```python
from build123d import *

# Parameters (mm, degrees)
BOSS_EXTRUDE1_DEPTH = 5.5118
SKETCH2_R           = 5.08
CUT_EXTRUDE1_DEPTH  = 2.286
BOSS_EXTRUDE2_DEPTH = 4.6228


with BuildPart() as part:
    # Sketch1 → Boss-Extrude1 (new body)
    with BuildSketch(Plane(origin=(0, 0, 0), x_dir=(1, 0, 0), z_dir=(0, 1, 0))):
        with BuildLine():
            ThreePointArc((20.407631134, 9.827266142), (20.718157649, 9.399980692), (20.828, 8.88332391))
            Line((20.828, 8.88332391), (20.828, -4.0386))
            Line((20.828, -4.0386), (24.257, -4.0386))
            Line((24.257, -4.0386), (24.257, -8.9916))
            ThreePointArc((24.257, -8.9916), (23.95942049, -9.71002049), (23.241, -10.0076))
            Line((23.241, -10.0076), (22.352, -10.0076))
            ThreePointArc((22.352, -10.0076), (21.274369265, -10.453969265), (20.828, -11.5316))
            Line((20.828, -11.5316), (20.828, -18.5166))
            Line((20.828, -18.5166), (-20.828, -18.5166))
            Line((-20.828, -18.5166), (-20.828, -11.5316))
            ThreePointArc((-20.828, -11.5316), (-21.274369265, -10.453969265), (-22.352, -10.0076))
            Line((-22.352, -10.0076), (-23.241, -10.0076))
            ThreePointArc((-23.241, -10.0076), (-23.95942049, -9.71002049), (-24.257, -8.9916))
            Line((-24.257, -8.9916), (-24.257, -4.0386))
            Line((-24.257, -4.0386), (-20.828, -4.0386))
            Line((-20.828, -4.0386), (-20.828, 8.88332391))
            ThreePointArc((-20.828, 8.88332391), (-20.718157649, 9.399980692), (-20.407631134, 9.827266142))
            Line((-20.407631134, 9.827266142), (-11.478262268, 17.864484463))
            ThreePointArc((-11.478262268, 17.864484463), (-10.689047654, 18.347973709), (-9.779, 18.5166))
            Line((-9.779, 18.5166), (9.779, 18.5166))
            ThreePointArc((9.779, 18.5166), (10.689047654, 18.347973709), (11.478262268, 17.864484463))
            Line((11.478262268, 17.864484463), (20.407631134, 9.827266142))
        make_face()
    extrude(amount=BOSS_EXTRUDE1_DEPTH)

    # Sketch2 → Cut-Extrude1 (cut)
    with BuildSketch(Plane(origin=(0, 5.5118, 0), x_dir=(1, 0, 0), z_dir=(0, 1, 0))):
        with Locations(Location((-9.9695, 0.7366, 0), (0, 0, 270))):
            Circle(SKETCH2_R)
        with Locations(Location((9.9695, 0.7366, 0), (0, 0, 270))):
            Circle(SKETCH2_R)
    extrude(amount=-CUT_EXTRUDE1_DEPTH, mode=Mode.SUBTRACT)

    # Sketch3 → Boss-Extrude2 (add)
    with BuildSketch(Plane.XZ):
        with BuildLine():
            Line((10.795, -17.2466), (-10.795, -17.2466))
            Line((-10.795, -17.2466), (-20.045633867, -8.920214887))
            Line((-20.045633867, -8.920214887), (-20.045633867, 11.4554))
            ThreePointArc((-20.045633867, 11.4554), (0, 12.967759921), (20.045633867, 11.4554))
            Line((20.045633867, 11.4554), (20.045633867, -8.920214887))
            Line((20.045633867, -8.920214887), (10.795, -17.2466))
        make_face()
    extrude(amount=BOSS_EXTRUDE2_DEPTH)


solid = part.part
```
Build history of the part. All positions in model axes, mm. A direction names the side the tool comes from. Round coordinates to 2 decimals unless told otherwise and drop trailing zeros. Write each loop counter-clockwise with the first axis right and the second up, starting at its lowest first coordinate (ties: lowest second). Pieces come first, ordered by that corner, then holes. Notation, with made-up numbers: (42, -29) -> (100, -29) arc R14 ccw to (100, -13) -> close; hole circle Ø7 at (67, 11.25). An arc over 180 degrees is marked (long way). Put each result on its own line as item: value.
Item 1: Slice it at A-A, the plane y = -3.25. Give the cut face in (x, z) (3 decimals).
Here are the results:
outline: (-20.046, -8.92) -> (-10.795, -17.247) -> (10.795, -17.247) -> (20.046, -8.92) -> (20.046, 11.455) arc R133.604 ccw to (-20.046, 11.455) -> close
Item 2: Slice it at C-C, the plane z = -15.5. Give the cut face in (x, y), plus the area to 3 significant figures.
Here are the results:
outline: (-14.11, 0) -> (-12.74, 0) -> (-12.74, -4.62) -> (12.74, -4.62) -> (12.74, 0) -> (14.11, 0) -> (14.11, 5.51) -> (-14.11, 5.51) -> close
area: 273 mm^2
Item 3: Wall check: probe 1 along X at (y, z) = (4.5, -5); probe 2 along Y at (x, z) = (-20.5, 6); probe 3 along X at (y, z) = (-0.5, 9). Give the ranges that are in metal, low to high. Write a range as from..to.
Here are the results:
probe 1: x = -20.83..-12.73, -7.21..7.21, 12.73..20.83
probe 2: y = 0..5.51
probe 3: x = -20.05..20.05
Item 4: Slice it at D-D, the plane y = 4. Give the cut face in (x, z), plus the area to 3 significant figures.
Here are the results:
outline: (-24.26, 4.04) -> (-20.83, 4.04) -> (-20.83, -8.88) arc R1.27 ccw to (-20.41, -9.83) -> (-11.48, -17.86) arc R2.54 ccw to (-9.78, -18.52) -> (9.78, -18.52) arc R2.54 ccw to (11.48, -17.86) -> (20.41, -9.83) arc R1.27 ccw to (20.83, -8.88) -> (20.83, 4.04) -> (24.26, 4.04) -> (24.26, 8.99) arc R1.02 ccw to (23.24, 10.01) -> (22.35, 10.01) arc R1.52 cw to (20.83, 11.53) -> (20.83, 18.52) -> (-20.83, 18.52) -> (-20.83, 11.53) arc R1.52 cw to (-22.35, 10.01) -> (-23.24, 10.01) arc R1.02 ccw to (-24.26, 8.99) -> close; hole circle Ø10.16 at (-9.97, -0.74); hole circle Ø10.16 at (9.97, -0.74)
area: 1,330 mm^2
Item 5: Slice it at B-B, the plane x = -5.5. Give the cut face in (y, z).
Here are the results:
outline: (-4.62, -17.25) -> (0, -17.25) -> (0, -18.52) -> (5.51, -18.52) -> (5.51, -3.15) -> (3.23, -3.15) -> (3.23, 1.68) -> (5.51, 1.68) -> (5.51, 18.52) -> (0, 18.52) -> (0, 12.85) -> (-4.62, 12.85) -> close
Item 6: Tool access for faces 1 (the face through (-0.282, -2.279, 12.967)), 2 (the face through (15.485, -2.279, -13.025)), 3 (the face through (2, 0, 14)): list every direction of +Z, -Z, +X, -X, +Y, -Y with a clear straight run to the whole face (end or side of a thin tool).
Here are the results:
face 1: +Z, -Y
face 2: -Z, +X, -Y
face 3: -Y
Item 7: Flat gauge pins, fed straight in: P1, Ø4, axis at y = -1.5, z = -10.5, coming from the +X side; P2, Ø6, axis at x = -18.5, y = 0, coming from the -Z side; P3, Ø4.5, axis at y = 2, z = -2.5, coming from the -X side. Where does each tip first touch, or does it go through?
Here are the results:
P1: stops at x = 20.79
P2: stops at z = -14.24
P3: stops at x = -20.83
